Geometry: see drawing. Coordinates: mm, zero at the bounding-box minimum. A direction names the side the tool comes from. Coordinates: 2 decimals unless noted, no trailing zeros. Loops run counter-clockwise (first coordinate to the right, second up) from the corner with the lowest first, then second, coordinate; pieces in that order, holes last. Notation, with made-up numbers: (19, -33) - (74, -33) arc R14 cw to (74, -18) - close; hole circle Ø9 at (-5, 8). An arc over 180 degrees is marked (long way). Use a Markdown table: item, result. Add a question column.
1. Section query C-C on x = 28. Return the cut outline in (y, z), then the cut area to 3 significant figures.
2. Ray query, L1, parallel to Y at x = 93, z = 265; L2, parallel to Y at x = 42.5, z = 51.5; L3, parallel to Y at x = 44.5, z = 256.5. Return the intervals inside material, ascending. Write a range as [from, to].
3. Access query for the marked faces 1, 2 and 3. Directions: +Z, -Z, +X, -X, +Y, -Y. A direction counts if a zero-diameter tool reaches every point of the face in a straight line with its end or side. Return the directions, or none.
4. Contact query for flat-ended pins moving along their axis: P1, Ø8, axis at x = 67.5, z = 293.5, coming from the -Y side; P2, Ø1.5, axis at x = 49, z = 166, coming from the -Y side; P3, Ø1.5, axis at x = 21.5, y = 182.5, coming from the +Z side. Output: stop coordinate, or through.
5. Section query D-D on z = 368. Return the cut outline in (x, y), then the cut area to 3 significant figures.
6. Section query A-A on z = 265. Return the cut outline in (x, y).
7. Section query B-B on y = 1145. Return the cut outline in (x, z).
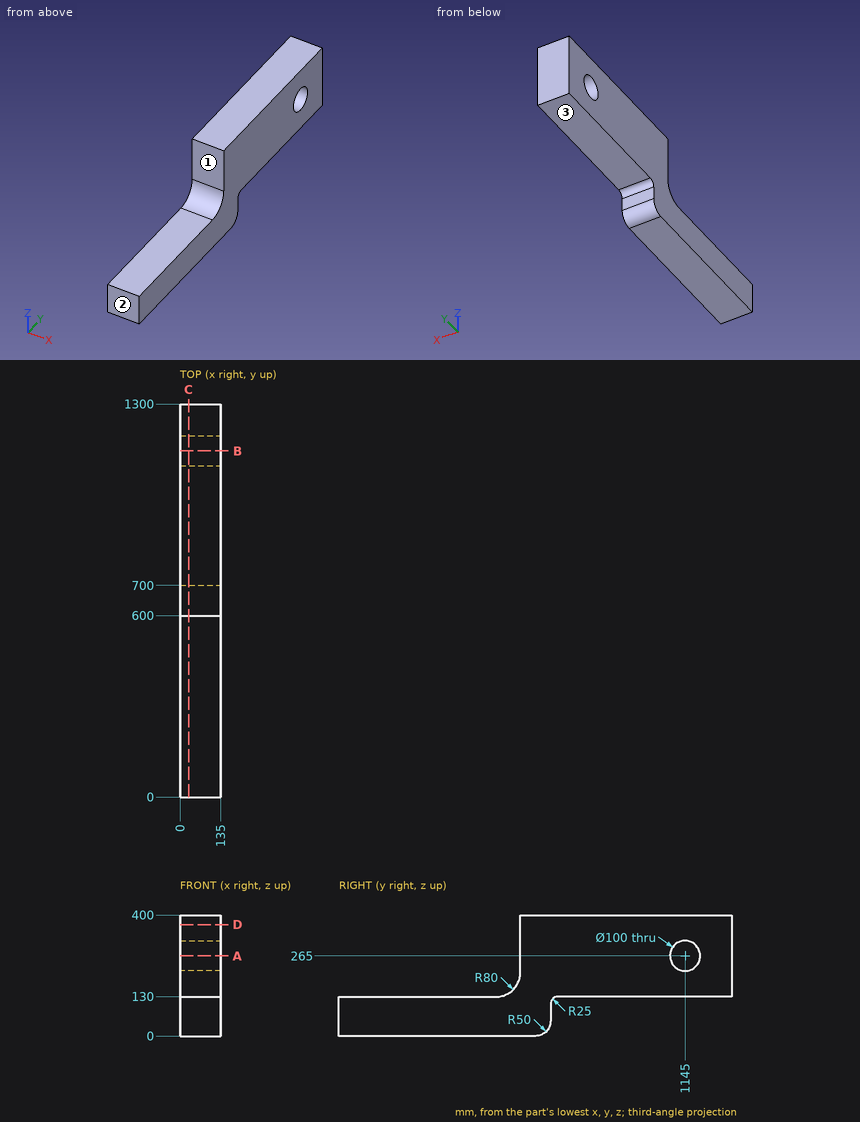
Resolved:
| question | item | result |
|---|---|---|
| 1 | outline | (0, 0) - (650, 0) arc R50 ccw to (700, 50) - (700, 105) arc R25 cw to (725, 130) - (1300, 130) - (1300, 400) - (600, 400) - (600, 210) arc R80 cw to (520, 130) - (0, 130) - close; hole circle Ø100 at (1145, 265) |
| 1 | area | 273,000 mm² |
| 2 | L1 | [600, 1095], [1195, 1300] |
| 2 | L2 | [0, 700] |
| 2 | L3 | [600, 1095.73], [1194.27, 1300] |
| 3 | face 1 | +Z, +X, -X, -Y |
| 3 | face 2 | +Z, -Z, +X, -X, -Y |
| 3 | face 3 | -Z, +X, -X, +Y |
| 4 | P1 | y = 600 |
| 4 | P2 | y = 586.31 |
| 4 | P3 | z = 130 |
| 5 | outline | (0, 600) - (135, 600) - (135, 1300) - (0, 1300) - close |
| 5 | area | 94,500 mm² |
| 6 | outline | (0, 600) - (135, 600) - (135, 1095) - (0, 1095) - close; (0, 1195) - (135, 1195) - (135, 1300) - (0, 1300) - close |
| 7 | outline | (0, 130) - (135, 130) - (135, 215) - (0, 215) - close; (0, 315) - (135, 315) - (135, 400) - (0, 400) - close |
